Build history of the part. All positions in model axes, mm. A direction names the side the tool comes from. Give positions to 0.01 mm unless a question says otherwise; leave off trailing zeros. Write each loop counter-clockwise with the first axis right and the second up, starting at its lowest first coordinate (ties: lowest second). Pieces come first, ordered by that corner, then holes. Notation, with made-up numbers: M 57,17.5 L 110,17.5 A26 ccw 110,34.5 Z; hole C 16.25,-12 d1. An arc over 180 degrees is marked long. Return JSON: item names as keys, results as strings. Group by question number.
Q1. Band-saw the part on A-A, the plane x = 3. Give the cut face in (y, z), then the cut area to 3 significant figures.
Q2. Flat gauge pins, fed straight in: pin 1 Ø1 at (x, z) = (-3, 24.5) entering from -Y; pin 2 Ø0.8 at (x, y) = (-1, 1) entering from +Z. Where does each tip first touch, or does it go through?
Q3. Band-saw the part on D-D, the plane z = -7. Give the cut face in (x, y), then the cut area to 3 significant figures.
Q4. Pull direction Z, two halves, no side cores. Call faces 1 (the flat face through (0, 1.5, 2)), 2 (the flat face through (3, 0.1, 18)), 3 (the cylindrical face through (22.85, 0.74, 23.11)): +Z half, -Z half, draft (parallel to the pull), parting line (faces both ways), or undercut.
Q5. Band-saw the part on B-B, the plane y = 0.7. Give the cut face in (x, z).
Q6. Wall check: probe 1 along X at (y, z) = (1.2, -22); probe 2 along X at (y, z) = (1.3, 7); probe 3 along Z at (x, y) = (-4, 1). Give the ranges that are in metal, low to high.
Q7. Tool access for faces 4 (the cylindrical face through (-21.673, 0.74, -20.105)), 5 (the flat face through (27.203, 1, 0)), 6 (the flat face through (-3, 0.1, 21)), 7 (the flat face through (-27.203, 1, 0)), 8 (the flat face through (-12, 1, 29)): list every direction of +Z, -Z, +X, -X, +Y, -Y with a clear straight run to the whole face (end or side of a thin tool).
Q8. Band-saw the part on C-C, the plane z = -16.5. Give the cut face in (x, y), then the cut area to 3 significant figures.
from build123d import *

# Parameters (mm, degrees)
SKETCH_1_R          = 32.5
SKETCH_1_R_2        = 1.2
EXTRUDE_1_DEPTH     = 1.5
CUT_EXTRUDE_1_DEPTH = 46.986411036
CUT_EXTRUDE_2_DEPTH = 43.74049602
SKETCH_4_R          = 1.5
SKETCH_4_R_2        = 1
CUT_EXTRUDE_3_DEPTH = 0.1


with BuildPart() as part:
    # 草图1 → 凸台-拉伸1 (new body)
    with BuildSketch(Plane(origin=(0, 0, 0), x_dir=(1, 0, 0), z_dir=(0, 1, 0))):
        with Locations(Location((0, 0, 0), (0, 0, 270))):
            Circle(SKETCH_1_R)
        with Locations(Location((21.213203436, 21.213203436, 0), (0, 0, 270))):
            Circle(SKETCH_1_R_2, mode=Mode.SUBTRACT)
        with Locations(Location((21.213203436, -21.213203436, 0), (0, 0, 270))):
            Circle(SKETCH_1_R_2, mode=Mode.SUBTRACT)
        with Locations(Location((-21.213203436, -21.213203436, 0), (0, 0, 270))):
            Circle(SKETCH_1_R_2, mode=Mode.SUBTRACT)
        with Locations(Location((-21.213203436, 21.213203436, 0), (0, 0, 270))):
            Circle(SKETCH_1_R_2, mode=Mode.SUBTRACT)
    extrude(amount=EXTRUDE_1_DEPTH)

    # 草图2 → 切除-拉伸1 (cut, through all)
    with BuildSketch(Plane(origin=(0, 1.5, 0), x_dir=(1, 0, 0), z_dir=(0, 1, 0))):
        with BuildLine():
            Line((30.203476621, 12), (27.203476621, 12))
            Line((27.203476621, 12), (27.203476621, -12))
            Line((27.203476621, -12), (30.203476621, -12))
            ThreePointArc((30.203476621, -12), (32.5, 0), (30.203476621, 12))
        make_face()
        with BuildLine():
            Line((12, -27.203476621), (-12, -27.203476621))
            Line((-12, -27.203476621), (-12, -30.203476621))
            ThreePointArc((-12, -30.203476621), (0, -32.5), (12, -30.203476621))
            Line((12, -30.203476621), (12, -27.203476621))
        make_face()
        with BuildLine():
            Line((-27.203476621, -12), (-27.203476621, 12))
            Line((-27.203476621, 12), (-30.203476621, 12))
            ThreePointArc((-30.203476621, 12), (-32.5, 0), (-30.203476621, -12))
            Line((-30.203476621, -12), (-27.203476621, -12))
        make_face()
        with BuildLine():
            Line((-12, 27.203476621), (12, 27.203476621))
            Line((12, 27.203476621), (12, 30.203476621))
            ThreePointArc((12, 30.203476621), (0, 32.5), (-12, 30.203476621))
            Line((-12, 30.203476621), (-12, 27.203476621))
        make_face()
    extrude(amount=-CUT_EXTRUDE_1_DEPTH, mode=Mode.SUBTRACT)

    # 草图3 → 切除-拉伸2 (cut, through all)
    with BuildSketch(Plane(origin=(0, 1.5, 0), x_dir=(1, 0, 0), z_dir=(0, 1, 0))):
        Polygon((17, 26.25), (-17, 26.25), (-27.149655647, 26.25), (-14.240374978, 46.745445694), (28.149411973, 26.25), align=None)
    extrude(amount=-CUT_EXTRUDE_2_DEPTH, mode=Mode.SUBTRACT)

    # 草图4 → 切除-拉伸3 (cut)
    with BuildSketch(Plane.XZ):
        with Locations(Location((3, 22.203476621, 0), (0, 0, 270))):
            Circle(SKETCH_4_R)
        with Locations(Location((3, 18.203476621, 0), (0, 0, 270))):
            Circle(SKETCH_4_R)
        with Locations(Location((-6, 24.203476621, 0), (0, 0, 270))):
            Circle(SKETCH_4_R_2)
        with Locations(Location((-3, 24.203476621, 0), (0, 0, 270))):
            Circle(SKETCH_4_R_2)
        with Locations(Location((-3, 21.203476621, 0), (0, 0, 270))):
            Circle(SKETCH_4_R_2)
        with Locations(Location((-6, 21.203476621, 0), (0, 0, 270))):
            Circle(SKETCH_4_R_2)
    extrude(amount=-CUT_EXTRUDE_3_DEPTH, mode=Mode.SUBTRACT)


solid = part.part
From the geometry:
{
 "1": {"outline": "M 0,-26.25 L 1.5,-26.25 L 1.5,27.2 L 0,27.2 L 0,23.7 L 0.1,23.7 L 0.1,20.7 L 0,20.7 L 0,19.7 L 0.1,19.7 L 0.1,16.7 L 0,16.7 Z", "area": "79.6 mm^2"},
 "2": {"pin 1": "stops at y = 0.1", "pin 2": "stops at z = 27.2"},
 "3": {"outline": "M -27.2,0 L 27.2,0 L 27.2,1.5 L -27.2,1.5 Z", "area": "81.6 mm^2"},
 "4": {"face 1": "draft", "face 2": "undercut", "face 3": "+Z half"},
 "5": {"outline": "M -30.2,-12 A32.5 ccw -19.16,-26.25 L 19.16,-26.25 A32.5 ccw 30.2,-12 L 27.2,-12 L 27.2,12 L 30.2,12 A32.5 ccw 12,30.2 L 12,27.2 L -12,27.2 L -12,30.2 A32.5 ccw -30.2,12 L -27.2,12 L -27.2,-12 Z; hole C -21.21,-21.21 d2.4; hole C -21.21,21.21 d2.4; hole C 21.21,-21.21 d2.4; hole C 21.21,21.21 d2.4"},
 "6": {"probe 1": "x = -23.92 to -22.12, -20.31 to 20.31, 22.12 to 23.92", "probe 2": "x = -27.2 to 27.2", "probe 3": "z = -26.25 to 27.2"},
 "7": {"face 4": "+Y, -Y", "face 5": "+X, +Y, -Y", "face 6": "-Y", "face 7": "-X, +Y, -Y", "face 8": "+Z, +Y, -Y"},
 "8": {"outline": "M -28,0 L 28,0 L 28,1.5 L -28,1.5 Z", "area": "84.0 mm^2"}
}
